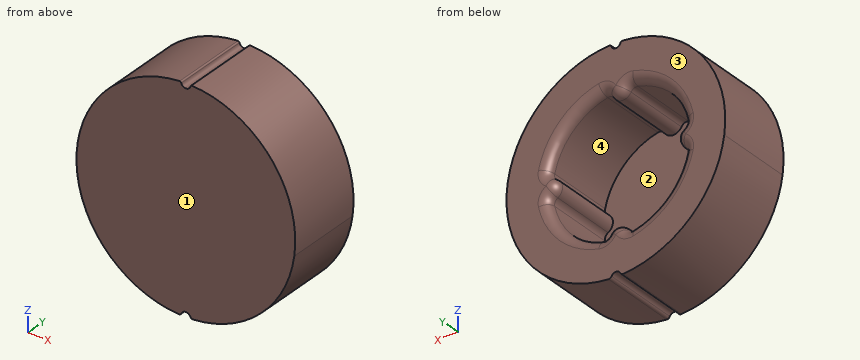
```python
from build123d import *

# Parameters (mm, degrees)
BOSS_EXTRUDE1_DEPTH = 25
CUT_EXTRUDE2_DEPTH  = 26
BOSS_EXTRUDE2_DEPTH = 0.4
FILLET1_R           = 3


with BuildPart() as part:
    # Sketch1 → Boss-Extrude1 (new body)
    with BuildSketch(Plane(origin=(0, 0, 0), x_dir=(1, 0, 0), z_dir=(0, 1, 0))):
        with BuildLine():
            ThreePointArc((1.451818925, -34.068556857), (1.641248992, -34.346908706), (1.964225605, -34.442038138))
            ThreePointArc((1.964225605, -34.442038138), (26.591847487, -21.978073076), (34.198225299, 4.555174015))
            ThreePointArc((34.198225299, 4.555174015), (23.590291339, 25.176355888), (2.324135821, 34.423627607))
            ThreePointArc((2.324135821, 34.423627607), (1.751838249, 34.289058819), (1.354061739, 33.856153382))
            ThreePointArc((1.354061739, 33.856153382), (0, 33.001534515), (-1.354061739, 33.856153382))
            ThreePointArc((-1.354061739, 33.856153382), (-1.751838249, 34.289058819), (-2.324135821, 34.423627607))
            ThreePointArc((-2.324135821, 34.423627607), (-23.590291339, 25.176355888), (-34.198225299, 4.555174015))
            ThreePointArc((-34.198225299, 4.555174015), (-26.591847487, -21.978073076), (-1.964225605, -34.442038138))
            ThreePointArc((-1.964225605, -34.442038138), (-1.641248992, -34.346908706), (-1.451818925, -34.068556857))
            ThreePointArc((-1.451818925, -34.068556857), (0, -32.945679925), (1.451818925, -34.068556857))
        make_face()
        with BuildLine():
            Line((-2.417, 3.787737139), (0, 3.787737139))
            Line((0, 3.787737139), (2.417, 3.787737139))
            ThreePointArc((2.417, 3.787737139), (0, -4.489512172), (-2.417, 3.787737139))
        make_face(mode=Mode.SUBTRACT)
    extrude(amount=BOSS_EXTRUDE1_DEPTH)

    # Sketch2 → Cut-Extrude2 (cut, through all)
    with BuildSketch(Plane(origin=(0, 0, 0), x_dir=(1, 0, 0), z_dir=(0, 1, 0))):
        with BuildLine():
            ThreePointArc((-21.475, -4.777486264), (-15.556349186, -15.556349186), (-4.777486264, -21.475))
            ThreePointArc((-4.777486264, -21.475), (-3.533555097, -21.35153147), (-2.605901598, -20.513636364))
            ThreePointArc((-2.605901598, -20.513636364), (0, -19), (2.605901598, -20.513636364))
            ThreePointArc((2.605901598, -20.513636364), (3.533555097, -21.35153147), (4.777486264, -21.475))
            ThreePointArc((4.777486264, -21.475), (15.556349186, -15.556349186), (21.475, -4.777486264))
            ThreePointArc((21.475, -4.777486264), (21.35153147, -3.533555097), (20.513636364, -2.605901598))
            ThreePointArc((20.513636364, -2.605901598), (19, 0), (20.513636364, 2.605901598))
            ThreePointArc((20.513636364, 2.605901598), (21.35153147, 3.533555097), (21.475, 4.777486264))
            ThreePointArc((21.475, 4.777486264), (15.556349186, 15.556349186), (4.777486264, 21.475))
            ThreePointArc((4.777486264, 21.475), (3.533555097, 21.35153147), (2.605901598, 20.513636364))
            ThreePointArc((2.605901598, 20.513636364), (0, 19), (-2.605901598, 20.513636364))
            ThreePointArc((-2.605901598, 20.513636364), (-3.533555097, 21.35153147), (-4.777486264, 21.475))
            ThreePointArc((-4.777486264, 21.475), (-15.556349186, 15.556349186), (-21.475, 4.777486264))
            ThreePointArc((-21.475, 4.777486264), (-21.35153147, 3.533555097), (-20.513636364, 2.605901598))
            ThreePointArc((-20.513636364, 2.605901598), (-19, 0), (-20.513636364, -2.605901598))
            ThreePointArc((-20.513636364, -2.605901598), (-21.35153147, -3.533555097), (-21.475, -4.777486264))
        make_face()
    extrude(amount=CUT_EXTRUDE2_DEPTH, mode=Mode.SUBTRACT)

    # Sketch2<2> → Boss-Extrude2 (add)
    with BuildSketch(Plane(origin=(0, 0, 0), x_dir=(1, 0, 0), z_dir=(0, 1, 0))):
        with BuildLine():
            ThreePointArc((-21.475, -4.777486264), (-15.556349186, -15.556349186), (-4.777486264, -21.475))
            ThreePointArc((-4.777486264, -21.475), (-3.533555097, -21.35153147), (-2.605901598, -20.513636364))
            ThreePointArc((-2.605901598, -20.513636364), (0, -19), (2.605901598, -20.513636364))
            ThreePointArc((2.605901598, -20.513636364), (3.533555097, -21.35153147), (4.777486264, -21.475))
            ThreePointArc((4.777486264, -21.475), (15.556349186, -15.556349186), (21.475, -4.777486264))
            ThreePointArc((21.475, -4.777486264), (21.35153147, -3.533555097), (20.513636364, -2.605901598))
            ThreePointArc((20.513636364, -2.605901598), (19, 0), (20.513636364, 2.605901598))
            ThreePointArc((20.513636364, 2.605901598), (21.35153147, 3.533555097), (21.475, 4.777486264))
            ThreePointArc((21.475, 4.777486264), (15.556349186, 15.556349186), (4.777486264, 21.475))
            ThreePointArc((4.777486264, 21.475), (3.533555097, 21.35153147), (2.605901598, 20.513636364))
            ThreePointArc((2.605901598, 20.513636364), (0, 19), (-2.605901598, 20.513636364))
            ThreePointArc((-2.605901598, 20.513636364), (-3.533555097, 21.35153147), (-4.777486264, 21.475))
            ThreePointArc((-4.777486264, 21.475), (-15.556349186, 15.556349186), (-21.475, 4.777486264))
            ThreePointArc((-21.475, 4.777486264), (-21.35153147, 3.533555097), (-20.513636364, 2.605901598))
            ThreePointArc((-20.513636364, 2.605901598), (-19, 0), (-20.513636364, -2.605901598))
            ThreePointArc((-20.513636364, -2.605901598), (-21.35153147, -3.533555097), (-21.475, -4.777486264))
        make_face()
    extrude(amount=BOSS_EXTRUDE2_DEPTH)

    # Fillet1
    fillet1_edges = [part.edges().sort_by_distance(p)[0] for p in [
        (-21.35153147, 25, 3.533555097),
        (-15.556349186, 25, 15.556349186),
        (-3.533555097, 25, 21.35153147),
        (0, 25, 19),
        (3.533555097, 25, 21.35153147),
        (15.556349186, 25, 15.556349186),
        (21.35153147, 25, 3.533555097),
        (19, 25, 0),
        (21.35153147, 25, -3.533555097),
        (15.556349186, 25, -15.556349186),
        (3.533555097, 25, -21.35153147),
        (0, 25, -19),
        (-3.533555097, 25, -21.35153147),
        (-15.556349186, 25, -15.556349186),
        (-21.35153147, 25, -3.533555097),
        (-19, 25, 0),
    ]]
    fillet(fillet1_edges, radius=FILLET1_R)


solid = part.part
```
The listing builds one solid part. Answer for the finished solid, in the listing's coordinates (mm). Face numbers are marked on the shaded views. A direction names the side the tool comes from. Round coordinates to 2 decimals unless told otherwise and drop trailing zeros. Order: outer loops, then holes, each group sorted by start corner. A loop starts at its lowest first (then second) coordinate and runs counter-clockwise, first axis right, second up. Notation, with made-up numbers: (84, 6.25) -> (96, 6.25) arc R24 ccw to (96, 19.25) -> close; hole circle Ø5 at (16, -26). An arc over 180 degrees is marked (long way). Answer as CSV lines item,"result". Start each with the question number.
(1) For a pull along X with two mould halves and no side action, classify the marked faces 3 and 4 as +X half, -X half, draft (parallel to the pull), parting line (faces both ways), or undercut.
(2) Find the intervals of material crossed by probe 1 along X at (y, z) = (4.75, 20); probe 2 along Z at (x, y) = (-6, 17.75); probe 3 along Z at (x, y) = (9, 11), in increasing order. Write a range as from..to.
(3) Flat-ended cylindrical pins translate along their axes: pin 1 Ø10 at (x, y) = (-16, 3) entering from -Z; pin 2 Ø21.5 at (x, z) = (0.5, -10) entering from +Y; pin 3 Ø12 at (x, y) = (-26.5, 9) entering from +Z. Find the tip coordinate at first contact, or state that the pin passes through.
(4) A tool of negligible diameter and unlimited length cuts with its end or side. For the marked faces 1 and 2, from which of +Z, -Z, +X, -X, +Y, -Y can it reach the whole face along a straight path? Write none if from no direction.
(5) The part is cut by section A-A (y = 2.75). Determine the outline of the cut face in (x, z) (3 decimals), then the cut area to 3 significant figures.
Evaluation:
1,face 3,"draft"
1,face 4,"undercut"
2,probe 1,"-28.11..-9.17, -2.24..2.24, 9.17..28.11"
2,probe 2,"-33.98..-21.17, 21.17..33.97"
2,probe 3,"-33.31..-20.07, 20.07..33.3"
3,pin 1,"z = -32.7"
3,pin 2,"y = 24.72"
3,pin 3,"z = 27.75"
4,face 1,"+Z, -Z, +X, -X, -Y"
4,face 2,"+Y"
5,outline,"(-2.324, -34.424) arc R1 ccw to (-1.354, -33.856) arc R1.5 cw to (1.354, -33.856) arc R1 ccw to (2.324, -34.424) arc R34.5 ccw to (1.964, 34.442) arc R0.5 ccw to (1.452, 34.069) arc R1.5 cw to (-1.452, 34.069) arc R0.5 ccw to (-1.964, 34.442) arc R34.5 ccw to start; hole (-21.475, -4.777) arc R22 ccw to (-4.777, -21.475) arc R2 ccw to (-2.606, -20.514) arc R3 cw to (2.606, -20.514) arc R2 ccw to (4.777, -21.475) arc R22 ccw to (21.475, -4.777) arc R2 ccw to (20.514, -2.606) arc R3 cw to (20.514, 2.606) arc R2 ccw to (21.475, 4.777) arc R22 ccw to (4.777, 21.475) arc R2 ccw to (2.606, 20.514) arc R3 cw to (-2.606, 20.514) arc R2 ccw to (-4.777, 21.475) arc R22 ccw to (-21.475, 4.777) arc R2 ccw to (-20.514, 2.606) arc R3 cw to (-20.514, -2.606) arc R2 ccw to start"
5,area,"2,270 mm²"
